from build123d import *

# Parameters (mm, degrees)
SKETCH1_W           = 32
SKETCH1_H           = 60
BOSS_EXTRUDE1_DEPTH = 24.2
SHELL1_T            = 3
SKETCH3_W           = 3
SKETCH3_H           = 32
CUT_EXTRUDE1_DEPTH  = 24.2
BOSS_EXTRUDE2_START = 24.2
SKETCH4_W           = 60
SKETCH4_H           = 78
BOSS_EXTRUDE2_DEPTH = 3
CUT_EXTRUDE2_DEPTH  = 3
SKETCH6_R           = 2.25
CUT_EXTRUDE3_DEPTH  = 3
FILLET2_R           = 10
FILLET3_R           = 10
FILLET4_R           = 10


with BuildPart() as part:
    # Sketch1 → Boss-Extrude1 (new body)
    with BuildSketch(Plane(origin=(0, 0, 0), x_dir=(0, 1, 0), z_dir=(0, 0, 1))):
        Rectangle(SKETCH1_W, SKETCH1_H)
    extrude(amount=BOSS_EXTRUDE1_DEPTH)

    # Shell1
    shell1_openings = [part.faces().sort_by_distance(p)[0] for p in [
        (0, 0, 24.2),
    ]]
    offset(amount=SHELL1_T, openings=shell1_openings, kind=Kind.INTERSECTION)

    # Sketch3 → Cut-Extrude1 (cut)
    with BuildSketch(Plane.XY.offset(24.2)):
        with Locations((31.5, 0)):
            Rectangle(SKETCH3_W, SKETCH3_H)
    extrude(amount=-CUT_EXTRUDE1_DEPTH, mode=Mode.SUBTRACT)

    # Sketch4 → Boss-Extrude2 (add)
    with BuildSketch(Plane(origin=(0, 0, 0), x_dir=(0, 1, 0), z_dir=(0, 0, 1)).offset(BOSS_EXTRUDE2_START)):
        with Locations((-0.351117191, 6)):
            Rectangle(SKETCH4_W, SKETCH4_H)
    extrude(amount=-BOSS_EXTRUDE2_DEPTH)

    # Sketch5 → Cut-Extrude2 (cut)
    with BuildSketch(Plane.XY.offset(24.2)):
        Polygon((-30, -16), (30, -16), (33, -16), (33, -32.34351268), (43.583685091, -32.34351268), (43.583685091, 31.729117596), (33, 31.729117596), (33, 16), (30, 16), (-30, 16), align=None)
    extrude(amount=-CUT_EXTRUDE2_DEPTH, mode=Mode.SUBTRACT)

    # Sketch6 → Cut-Extrude3 (cut)
    with BuildSketch(Plane(origin=(0, 0, 21.2), x_dir=(1, 0, 0), z_dir=(0, 0, -1))):
        with Locations(Location((-14.936067977, -27, 0), (0, 0, 180))):
            Circle(SKETCH6_R)
        with Locations(Location((-38.5, 19, 0), (0, 0, 180))):
            Circle(SKETCH6_R)
    extrude(amount=-CUT_EXTRUDE3_DEPTH, mode=Mode.SUBTRACT)

    # Fillet2
    # the kernel refuses this fillet: 10 mm, written as the material it takes off along each edge
    with BuildSketch(Plane(origin=(-33, 44, -3), x_dir=(1, 0, 0), z_dir=(0, -1, 0))) as fillet2_piece_1:
        with BuildLine():
            CenterArc((FILLET2_R, FILLET2_R), FILLET2_R, 180, 90)
            Line((0, FILLET2_R), (0, 0))
            Line((0, 0), (FILLET2_R, 0))
        make_face()
    extrude(amount=88, mode=Mode.SUBTRACT)
    with BuildSketch(Plane(origin=(-58, -19, -3), x_dir=(0, 0, 1), z_dir=(1, 0, 0)), Plane(origin=(58, 19, -3), x_dir=(0, 0, 1), z_dir=(-1, 0, 0))) as fillet2_piece_2:
        with BuildLine():
            CenterArc((FILLET2_R, -FILLET2_R), FILLET2_R, 90, 90)
            Line((0, -FILLET2_R), (0, 0))
            Line((0, 0), (FILLET2_R, 0))
        make_face()
    extrude(amount=116, mode=Mode.SUBTRACT)
    with BuildSketch(Plane(origin=(33, -44, -3), x_dir=(0, 0, 1), z_dir=(0, 1, 0))) as fillet2_piece_3:
        with BuildLine():
            CenterArc((FILLET2_R, -FILLET2_R), FILLET2_R, 90, 90)
            Line((0, -FILLET2_R), (0, 0))
            Line((0, 0), (FILLET2_R, 0))
        make_face()
    extrude(amount=88, mode=Mode.SUBTRACT)

    # Fillet3
    fillet3_edges = [part.edges().sort_by_distance(p)[0] for p in [
        (0.070714214, 16, 0),
        (-30, 0, 0),
        (0.070714214, -16, 0),
    ]]
    fillet(fillet3_edges, radius=FILLET3_R)

    # Fillet4
    # the kernel refuses this fillet: 10 mm, written as the material it takes off along each edge
    with BuildSketch(Plane(origin=(-23, 9, 7), x_dir=(0, 1, 0), z_dir=(-1, 0, 0))) as fillet4_piece_1_section:
        Polygon((0, 0), (FILLET4_R * 1.02, 0), (FILLET4_R * 1.02, FILLET4_R * 1.02), (0, FILLET4_R * 1.02), align=None)
    fillet4_piece_1 = extrude(amount=FILLET4_R * 1.02, mode=Mode.PRIVATE)
    fillet4_piece_1 = fillet4_piece_1 - Plane(origin=(-23, 9, 7), x_dir=(0, -0.7071067811865475, 0.7071067811865475), z_dir=(-1, 0, 0)) * Sphere(FILLET4_R, mode=Mode.PRIVATE)
    add(fillet4_piece_1, mode=Mode.SUBTRACT)
    with BuildSketch(Plane(origin=(-23, -9, 7), x_dir=(-1, 0, 0), z_dir=(0, -1, 0))) as fillet4_piece_2_section:
        Polygon((0, 0), (FILLET4_R * 1.02, 0), (FILLET4_R * 1.02, FILLET4_R * 1.02), (0, FILLET4_R * 1.02), align=None)
    fillet4_piece_2 = extrude(amount=FILLET4_R * 1.02, mode=Mode.PRIVATE)
    fillet4_piece_2 = fillet4_piece_2 - Plane(origin=(-23, -9, 7), x_dir=(0.7071067811865475, 0, 0.7071067811865475), z_dir=(0, -1, 0)) * Sphere(FILLET4_R, mode=Mode.PRIVATE)
    add(fillet4_piece_2, mode=Mode.SUBTRACT)
    with BuildSketch(Plane(origin=(-33, -19, 7), x_dir=(1, 0, 0), z_dir=(0, 0, 1)), Plane(origin=(-33, 19, 7), x_dir=(0, -1, 0), z_dir=(0, 0, 1))) as fillet4_piece_3:
        with BuildLine():
            CenterArc((FILLET4_R, FILLET4_R), FILLET4_R, 180, 90)
            Line((0, FILLET4_R), (0, 0))
            Line((0, 0), (FILLET4_R, 0))
        make_face()
    extrude(amount=14.2, mode=Mode.SUBTRACT)


solid = part.part
Here's how the part is built. I have some questions about the finished solid (model axes, mm). A direction names the side the tool comes from. Coordinates: 2 decimals unless noted, no trailing zeros. Loops run counter-clockwise (first coordinate to the right, second up) from the corner with the lowest first, then second, coordinate; pieces in that order, holes last.
1. Imagine slicing it at C-C, the plane z = 15.25. Please give me the cut outline in (x, y).
2. Imagine slicing it at A-A, the plane x = -38.5. Please give me the cut outline in (y, z).
3. For P1, Ø4.5, axis at y = 0, z = 14.5, coming from the +X side; P2, Ø6, axis at x = -31.5, y = 11, coming from the -Z side; P3, Ø3.5, axis at x = -5, y = -0.5, coming from the +Z side, each with a flat end and sliding along its axis, tell me the tip position at first contact or that it passes through.
4. Imagine slicing it at B-B, the plane y = 27. Please give me the cut outline in (x, z), and give its area (4 significant figures).
5. Imagine slicing it at D-D, the plane x = 7.5. Please give me the cut outline in (y, z).
6. For faces 1 (the cylindrical face through (-31, -15, 14)), 2 (the cylindrical face through (1.06, 13.15, 3.01)), 3 (the flat face through (5, 19, 14)), which set-ups out of +Z, -Z, +X, -X, +Y, -Y let a thin tool reach every point of the face, with its end or its side?
7. I need wall thicknesses on L1, parallel to Y at x = 19, z = 22.5; L2, parallel to Y at x = -38.5, z = 23.6; L3, parallel to Z at x = -1.5, y = -5.5. Which ranges of each line are inside material? Lowest first, please.
8. If we mould it in two halves opening along Y, with no side actions, what happens to faces 4 (the flat face through (5, 0, 0)), 5 (the cylindrical face through (5.39, 16.15, 0.01)), 6 (the flat face through (33, -18, 20))? For each: pulls with the +Y half, pulls with the -Y half, needs draft (parallel to the pull), parting line crosses it, or undercut.
Taken from the geometry:
1. outline: (-33, -9) arc R10 ccw to (-23, -19) - (33, -19) - (33, -16) - (-30, -16) - (-30, 16) - (33, 16) - (33, 19) - (-23, 19) arc R10 ccw to (-33, 9) - close
2. outline: (-30.35, 21.2) - (-21.25, 21.2) - (-21.25, 24.2) - (-30.35, 24.2) - close; (-16.75, 21.2) - (29.65, 21.2) - (29.65, 24.2) - (-16.75, 24.2) - close
3. P1: stops at x = -30
3. P2: stops at z = -1.19
3. P3: stops at z = 0
4. outline: (-45, 21.2) - (-17.19, 21.2) - (-17.19, 24.2) - (-45, 24.2) - close; (-12.69, 21.2) - (33, 21.2) - (33, 24.2) - (-12.69, 24.2) - close
4. area: 220.5 mm2
5. outline: (-30.35, 21.2) - (-19, 21.2) - (-19, 7) arc R10 ccw to (-9, -3) - (9, -3) arc R10 ccw to (19, 7) - (19, 21.2) - (29.65, 21.2) - (29.65, 24.2) - (16, 24.2) - (16, 10) arc R10 cw to (6, 0) - (-6, 0) arc R10 cw to (-16, 10) - (-16, 24.2) - (-30.35, 24.2) - close
6. face 1: -Z, -X, -Y
6. face 2: +Z, +X
6. face 3: -Z, +X, -X, +Y
7. L1: y = -30.35 to -16, 16 to 29.65
7. L2: y = -30.35 to -21.25, -16.75 to 29.65
7. L3: z = -3 to 0
8. face 4: undercut
8. face 5: pulls with the +Y half
8. face 6: needs draft
